For this review, use the dimensioned drawing (mm, ordinates from the lowest corner) and the shaded views. Round coordinates to 2 decimals unless told otherwise and drop trailing zeros. Loops run counter-clockwise (first coordinate to the right, second up) from the corner with the lowest first, then second, coordinate; pieces in that order, holes last.
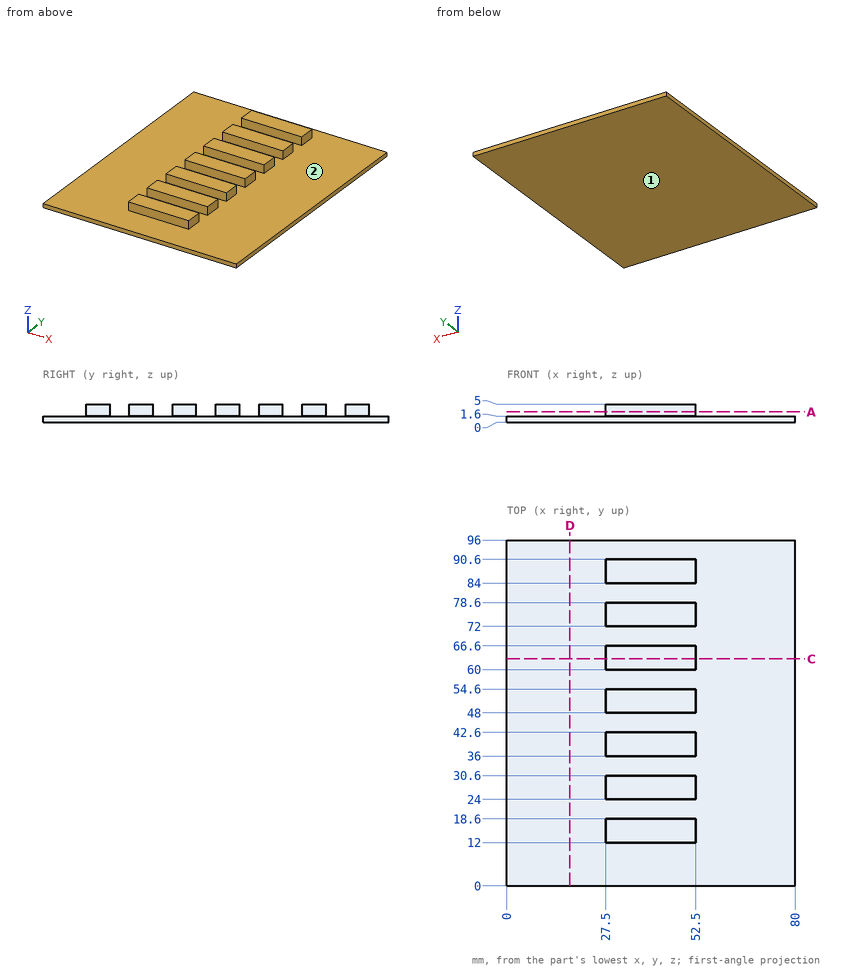
(1) For L1, parallel to Z at x = 26, y = 34; L2, parallel to X at y = 76, z = 1.7, list the stretches that pass through material, from the lowest coordinate up.
(2) Add section D-D (x = 17.5). Give the boundary of the cut face in (y, z), plus the area to 3 significant figures.
(3) Insertion check: pin 1 Ø1.7 at (x, z) = (44.5, 3) entering from +Y; pin 2 Ø1 at (y, z) = (86.5, 4) entering from +X; pin 3 Ø1 at (x, z) = (38, 3) entering from -Y. Each pin has a flat end and moves straight along its axis. Give the tip position at first contact, or say it passes through.
(4) Add section A-A (z = 2.8). Give the boundary of the cut face in (x, y).
(5) Add section C-C (y = 63). Give the boundary of the cut face in (x, z), plus the area to 3 significant figures.
(6) The part is to be moulded in two halves that separate along Y. For the marked faces 1 and 2, say which applies: pulls with the +Y half, pulls with the -Y half, needs draft (parallel to the pull), parting line crosses it, or undercut.
Outcome:
1. L1: z = 0 to 1.6
1. L2: x = 27.5 to 52.5
2. outline: (0, 0) - (96, 0) - (96, 1.6) - (0, 1.6) - close
2. area: 154 mm2
3. pin 1: stops at y = 90.6
3. pin 2: stops at x = 52.5
3. pin 3: stops at y = 12
4. outline: (27.5, 12) - (52.5, 12) - (52.5, 18.6) - (27.5, 18.6) - close; (27.5, 24) - (52.5, 24) - (52.5, 30.6) - (27.5, 30.6) - close; (27.5, 36) - (52.5, 36) - (52.5, 42.6) - (27.5, 42.6) - close; (27.5, 48) - (52.5, 48) - (52.5, 54.6) - (27.5, 54.6) - close; (27.5, 60) - (52.5, 60) - (52.5, 66.6) - (27.5, 66.6) - close; (27.5, 72) - (52.5, 72) - (52.5, 78.6) - (27.5, 78.6) - close; (27.5, 84) - (52.5, 84) - (52.5, 90.6) - (27.5, 90.6) - close
5. outline: (0, 0) - (80, 0) - (80, 1.6) - (52.5, 1.6) - (52.5, 5) - (27.5, 5) - (27.5, 1.6) - (0, 1.6) - close
5. area: 213 mm2
6. face 1: needs draft
6. face 2: undercut
